Here's how the part is built. I have some questions about the finished solid (model axes, mm). Face numbers are marked on the shaded views. Coordinates: 2 decimals unless noted, no trailing zeros. Use CSV: the item, a comma, the result in double quotes. Start each with the question number.
Q1. If we mould it in two halves opening along X, with no side actions, what happens to the marked faces 1 and 2? For each: +X half, -X half, draft (parallel to the pull), parting line (faces both ways), or undercut.
Q2. For pin 1 Ø3 at (y, z) = (17, 5.5) entering from +X; pin 2 Ø0.7 at (y, z) = (13, 0) entering from -X; pin 3 Ø1.1 at (x, z) = (0, -0.5) entering from -Y, each with a flat end and sliding along its axis, tell me the tip position at first contact or that it passes through.
Q3. Please list where these lines run through material, in increasing order: probe 1 along Z at (x, y) = (0, 13.5); probe 2 along Z at (x, y) = (0.25, 13.75); probe 3 along Z at (x, y) = (-4, 12). Write a range as [from, to].
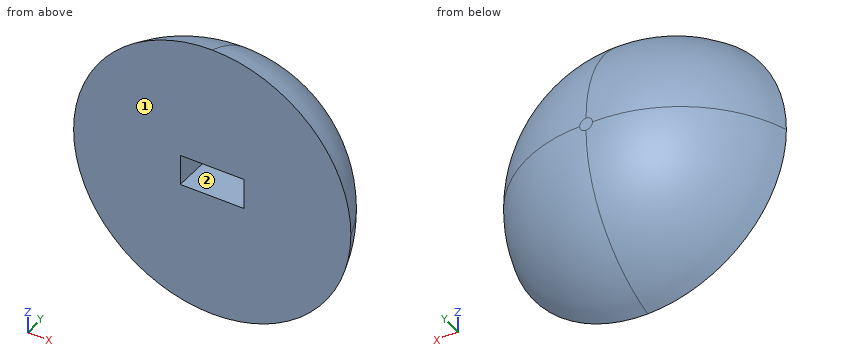
Autodesk Inventor part; units mm, degrees
ref_plane "YZ Plane" through (0, 0, 0) normal (1, 0, 0) x (0, 1, 0)
ref_plane "XZ Plane" through (0, 0, 0) normal (0, 1, 0) x (-1, 0, 0)
ref_plane "XY Plane" through (0, 0, 0) normal (0, 0, 1) x (1, 0, 0)
sketch "スケッチ1" plane through (0, 0, 0) normal (0, 0, 1) x (1, 0, 0)
  line L0 (2, 8) -> (-2, 8) construction
  line L1 (2, 8) -> (2, 13.5) construction
  line L2 (-2, 13.5) -> (2, 13.5) construction
  line L3 (-2, 8) -> (-2, 13.5) construction
  line L4 (-10, 8) -> (10, 8)
  line L5 (10, 8) -> (10, 18)
  line L6 (10, 18) -> (-10, 18)
  line L7 (-10, 18) -> (-10, 8)
  line L8 (0, -3.6) -> (0, 21.6) construction
  line L9 (-2.3, 13.8) -> (-2.3, 8)
  line L10 (-2.3, 13.8) -> (2.3, 13.8)
  line L11 (2.3, 13.8) -> (2.3, 8)
  line L12 (-10, 11) -> (10, 11)
  line L13 (-10, 14.5) -> (10, 14.5) construction
  point P0 (0, 0)
  point P1 (0, 18)
  point P2 (-2.3, 11)
  point P3 (2.3, 11)
  dimension "d0" = 20
  dimension "d1" = 10
  dimension "d2" = 0.3
  dimension "d3" = 0.3
  dimension "d4" = 0.3
  dimension "d5" = 3
  dimension "d6" = 3.5
extrude "押し出し1" add sketch "スケッチ1" along normal mid plane 20 contours L7 L6 L5 L12 L11 L10 L9 | L9 L10 L11 L12
extrude "押し出し2" cut sketch "スケッチ1" along normal mid plane 2.2 contours L9 L10 L11 L12
fillet "フィレット1" radius 10 4 edges at (-10, 14.5, 10) (-10, 14.5, -10) (10, 14.5, -10) (10, 14.5, 10)
fillet "フィレット2" radius 10 3 edges at (0, 18, 10) (-7.0711, 18, 7.0711) (-10, 18, 0)
properties part number "nob_L"
Results below:
1,face 1,"draft"
1,face 2,"undercut"
2,pin 1,"x = 4.92"
2,pin 2,"x = -9.31"
2,pin 3,"y = 13.8"
3,probe 1,"[-8.81, -1.1], [1.1, 8.81]"
3,probe 2,"[-8.64, -1.1], [1.1, 8.64]"
3,probe 3,"[-8.76, 8.76]"
